Here's how the part is built. I have some questions about the finished solid (model axes, mm). A direction names the side the tool comes from. Give positions to 0.01 mm unless a question says otherwise; leave off trailing zeros. Order: outer loops, then holes, each group sorted by start corner. A loop starts at its lowest first (then second) coordinate and runs counter-clockwise, first axis right, second up. Notation, with made-up numbers: M -35,14.5 L -20,14.5 A24 ccw -20,53.5 Z; hole C 14.5,65.25 d6. An arc over 180 degrees is marked long. Use one line per item in the form item = value.
from build123d import *

# Parameters (mm, degrees)
SKETCH2_W           = 70.5
SKETCH2_H           = 80
BOSS_EXTRUDE1_DEPTH = 10
SKETCH5_W           = 10
SKETCH5_H           = 68
CUT_EXTRUDE2_DEPTH  = 10
SKETCH8_W           = 50.5
SKETCH8_H           = 30
BOSS_EXTRUDE3_DEPTH = 10


with BuildPart() as part:
    # Sketch2 → Boss-Extrude1 (new body)
    with BuildSketch(Plane.XY):
        with Locations((0, 40)):
            Rectangle(SKETCH2_W, SKETCH2_H)
    extrude(amount=BOSS_EXTRUDE1_DEPTH)

    # Sketch5 → Cut-Extrude2 (cut)
    with BuildSketch(Plane.XY.offset(10)):
        with Locations((20.25, 40)):
            Rectangle(SKETCH5_W, SKETCH5_H)
        with Locations((-20.25, 40)):
            Rectangle(SKETCH5_W, SKETCH5_H)
        with Locations((0, 40)):
            Rectangle(SKETCH5_W, SKETCH5_H)
    extrude(amount=-CUT_EXTRUDE2_DEPTH, mode=Mode.SUBTRACT)

    # Sketch8 → Boss-Extrude3 (add)
    with BuildSketch(Plane.XY.offset(10)):
        with Locations((0, 59)):
            Rectangle(SKETCH8_W, SKETCH8_H)
    extrude(amount=-BOSS_EXTRUDE3_DEPTH)


solid = part.part
Q1. I need wall thicknesses on L1, parallel to X at y = 12, z = 2.75; L2, parallel to Y at x = -0.5, z = 7. Which ranges of each line are inside material? Lowest first, please.
Found:
L1 = -35.25 to -25.25, -15.25 to -5, 5 to 15.25, 25.25 to 35.25
L2 = 0 to 6, 44 to 80
Q2. I want a section at B-B on x = 22.5. Write out the boundary of the cut face in (y, z).
Found:
outline = M 0,0 L 6,0 L 6,10 L 0,10 Z; M 44,0 L 80,0 L 80,10 L 44,10 Z
Q3. I want a section at A-A on z = 1. Write out the boundary of the cut face in (x, y), then the cut area to 3 significant figures.
Found:
outline = M -35.25,0 L 35.25,0 L 35.25,80 L -35.25,80 Z; hole M -25.25,6 L -15.25,6 L -15.25,44 L -25.25,44 Z; hole M -5,6 L 5,6 L 5,44 L -5,44 Z; hole M 15.25,6 L 25.25,6 L 25.25,44 L 15.25,44 Z
area = 4,500 mm²
Q4. Thinking about a two-plate mould opening in Y: for faces 1 (the face through (0, 80, 5)), 2 (the face through (15.25, 25, 5)), 3 (the face through (0, 0, 5)), which applies, +Y half, -Y half, draft (parallel to the pull), parting line (faces both ways), or undercut?
Found:
face_1 = +Y half
face_2 = undercut
face_3 = -Y half
Q5. I want a section at C-C on y = 20.5. Write out the boundary of the cut face in (x, z).
Found:
outline = M -35.25,0 L -25.25,0 L -25.25,10 L -35.25,10 Z; M -15.25,0 L -5,0 L -5,10 L -15.25,10 Z; M 5,0 L 15.25,0 L 15.25,10 L 5,10 Z; M 25.25,0 L 35.25,0 L 35.25,10 L 25.25,10 Z
Q6. On a 3-axis mill with a long thin cutter (end or side, diameter ignored), from which of +Z, -Z, +X, -X, +Y, -Y can I reach the whole of each face in a straight line? I mean faces 4 (the face through (-35.25, 39, 5)), 5 (the face through (0, 44, 5)). Say none if no direction works.
Found:
face_4 = +Z, -Z, -X, +Y, -Y
face_5 = +Z, -Z
